Read the model definition and answer for the solid it produces. Units are mm, in the model's axes. Coordinates: 2 decimals unless noted, no trailing zeros. Order: outer loops, then holes, each group sorted by start corner. A loop starts at its lowest first (then second) coordinate and runs counter-clockwise, first axis right, second up.
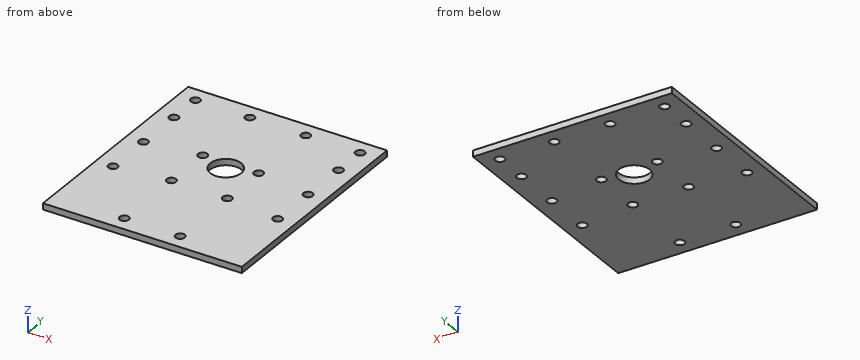
```python
from build123d import *

# Parameters (mm, degrees)
SKETCH1_W           = 64.001099834
SKETCH1_H           = 74
SKETCH1_R           = 1.5
SKETCH1_R_2         = 5
BOSS_EXTRUDE1_DEPTH = 2


with BuildPart() as part:
    # Sketch1 → Boss-Extrude1 (new body)
    with BuildSketch(Plane.XY):
        Rectangle(SKETCH1_W, SKETCH1_H)
        with Locations((-9, 8)):
            Circle(SKETCH1_R, mode=Mode.SUBTRACT)
        with Locations((26.5, -10)):
            Circle(SKETCH1_R, mode=Mode.SUBTRACT)
        with Locations((-9, 32)):
            Circle(SKETCH1_R, mode=Mode.SUBTRACT)
        with Locations((-9, -32)):
            Circle(SKETCH1_R, mode=Mode.SUBTRACT)
        with Locations((-9, -8)):
            Circle(SKETCH1_R, mode=Mode.SUBTRACT)
        with Locations((26.5, 5.5)):
            Circle(SKETCH1_R, mode=Mode.SUBTRACT)
        with Locations((26.5, 21)):
            Circle(SKETCH1_R, mode=Mode.SUBTRACT)
        with Locations((26.5, 32)):
            Circle(SKETCH1_R, mode=Mode.SUBTRACT)
        with Locations((9, 32)):
            Circle(SKETCH1_R, mode=Mode.SUBTRACT)
        with Locations((9, 8)):
            Circle(SKETCH1_R, mode=Mode.SUBTRACT)
        with Locations((9, -8)):
            Circle(SKETCH1_R, mode=Mode.SUBTRACT)
        with Locations((9, -32)):
            Circle(SKETCH1_R, mode=Mode.SUBTRACT)
        with Locations((-26.5, -10)):
            Circle(SKETCH1_R, mode=Mode.SUBTRACT)
        with Locations((-26.5, 5.5)):
            Circle(SKETCH1_R, mode=Mode.SUBTRACT)
        with Locations((-26.5, 21)):
            Circle(SKETCH1_R, mode=Mode.SUBTRACT)
        with Locations((-26.5, 32)):
            Circle(SKETCH1_R, mode=Mode.SUBTRACT)
        with Locations((0, 5.5)):
            Circle(SKETCH1_R_2, mode=Mode.SUBTRACT)
    extrude(amount=BOSS_EXTRUDE1_DEPTH)


solid = part.part
```
1) A cutting plane is placed at D-D, the plane y = -32. Determine the outline of the cut face in (x, z).
A:
outline: (-32, 0) - (-10.5, 0) - (-10.5, 2) - (-32, 2) - close; (-7.5, 0) - (7.5, 0) - (7.5, 2) - (-7.5, 2) - close; (10.5, 0) - (32, 0) - (32, 2) - (10.5, 2) - close
2) Flat-ended cylindrical pins translate along their axes: pin 1 Ø2.5 at (x, y) = (9, -32) entering from -Z; pin 2 Ø5 at (x, y) = (-9, -32) entering from -Z. Find the tip coordinate at first contact, or state that the pin passes through.
A:
pin 1: passes through
pin 2: stops at z = 0
3) A cutting plane is placed at B-B, the plane y = 32. Determine the outline of the cut face in (x, z), and give its area (3 significant figures).
A:
outline: (-32, 0) - (-28, 0) - (-28, 2) - (-32, 2) - close; (-25, 0) - (-10.5, 0) - (-10.5, 2) - (-25, 2) - close; (-7.5, 0) - (7.5, 0) - (7.5, 2) - (-7.5, 2) - close; (10.5, 0) - (25, 0) - (25, 2) - (10.5, 2) - close; (28, 0) - (32, 0) - (32, 2) - (28, 2) - close
area: 104 mm2
4) Straight lines are drawn through the part: line 1 (Y direction, x = -9, z = 1.2); line 2 (Y direction, x = -26.5, z = 1.5); line 3 (X direction, y = -32.5, z = 1.2). For each, find the intervals that lie inside material, in ascending order.
A:
line 1: y = -37 to -33.5, -30.5 to -9.5, -6.5 to 6.5, 9.5 to 30.5, 33.5 to 37
line 2: y = -37 to -11.5, -8.5 to 4, 7 to 19.5, 22.5 to 30.5, 33.5 to 37
line 3: x = -32 to -10.41, -7.59 to 7.59, 10.41 to 32
5) A cutting plane is placed at A-A, the plane x = 9. Determine the outline of the cut face in (y, z), and give its area (3 significant figures).
A:
outline: (-37, 0) - (-33.5, 0) - (-33.5, 2) - (-37, 2) - close; (-30.5, 0) - (-9.5, 0) - (-9.5, 2) - (-30.5, 2) - close; (-6.5, 0) - (6.5, 0) - (6.5, 2) - (-6.5, 2) - close; (9.5, 0) - (30.5, 0) - (30.5, 2) - (9.5, 2) - close; (33.5, 0) - (37, 0) - (37, 2) - (33.5, 2) - close
area: 124 mm2
6) A cutting plane is placed at C-C, the plane x = 0. Determine the outline of the cut face in (y, z).
A:
outline: (-37, 0) - (0.5, 0) - (0.5, 2) - (-37, 2) - close; (10.5, 0) - (37, 0) - (37, 2) - (10.5, 2) - close
